Verification items for this drawing (mm, ordinates from the low corner). Coordinates: 2 decimals unless noted, no trailing zeros. Order: outer loops, then holes, each group sorted by start corner. A loop starts at its lowest first (then second) coordinate and runs counter-clockwise, first axis right, second up. Notation, with made-up numbers: M 84.5,-7 L 92.5,-7 A4 ccw 92.5,0 Z; hole C -23,44 d6. An arc over 180 degrees is marked long. Answer as a JSON object with one key per item and string values. Group by question number.
(1) Cross-section at A-A (x = 30). Enter the section's corners in (y, z).
(2) Cross-section at C-C (y = 44). Enter the section's corners in (x, z), plus the area to 3 significant figures.
(3) Gauge pin test, flat ends, axial feed: pin 1 Ø2 at (y, z) = (28.5, 9.5) entering from -X; pin 2 Ø1.5 at (x, y) = (14, 39) entering from -Z; pin 3 Ø4 at (x, z) = (46, 21.5) entering from +Y. Record the tip position at first contact, or that the pin passes through.
(4) Material ranges on line 1 (Y direction, x = 30, z = 45); line 2 (Z direction, x = 50.5, y = 51); line 3 (Y direction, x = 19.5, z = 51) (1 decimal), recorded low to high.
(5) Cross-section at B-B (z = 21.5). Enter the section's corners in (x, y).
(6) Cross-section at D-D (x = 47.5). Enter the section's corners in (y, z) (1 decimal).
(7) Mould release check, pull along Y, two halves, no side actions. Record for the marked faces 1 and 2: released by +Y, released by -Y, zero draft, split by the parting line, or undercut.
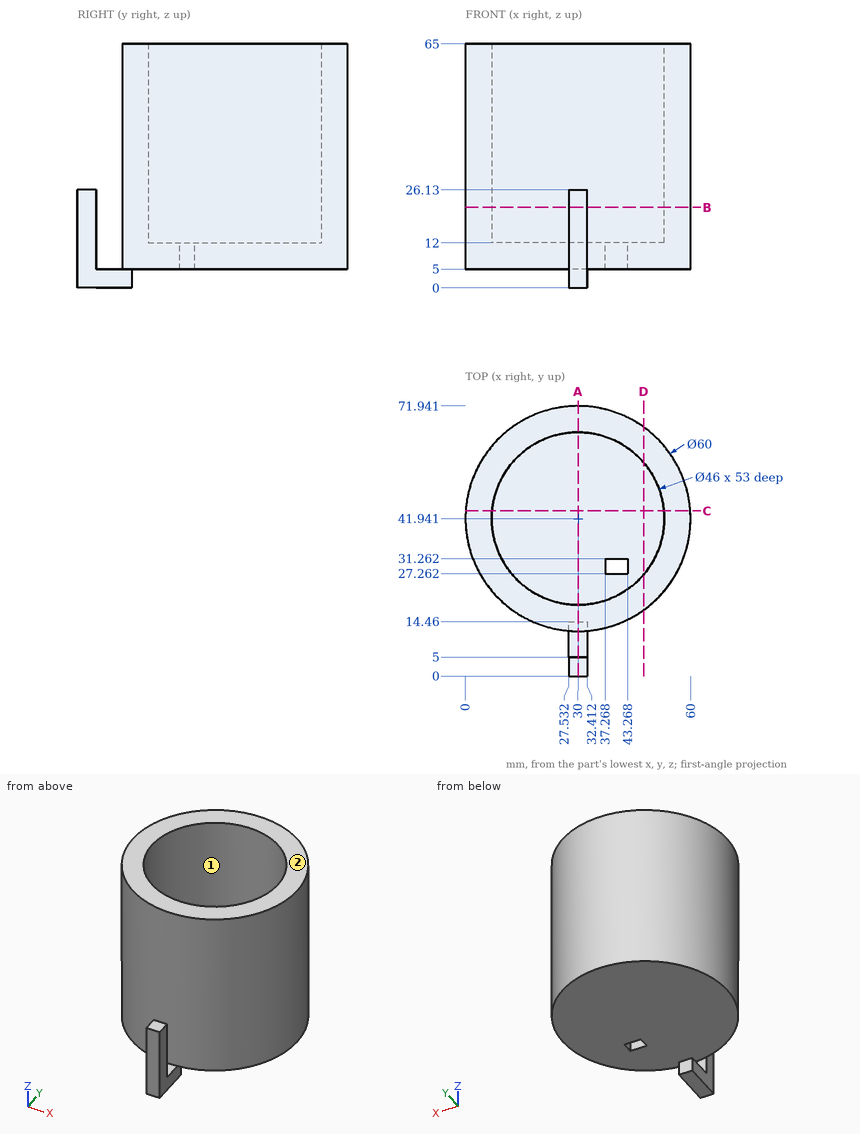
Taken from the geometry:
{
 "1": {"outline": "M 0,0 L 14.46,0 L 14.46,5 L 71.94,5 L 71.94,65 L 64.94,65 L 64.94,12 L 18.94,12 L 18.94,65 L 11.94,65 L 11.94,5 L 5,5 L 5,26.13 L 0,26.13 Z"},
 "2": {"outline": "M 0.07,5 L 59.93,5 L 59.93,65 L 52.91,65 L 52.91,12 L 7.09,12 L 7.09,65 L 0.07,65 Z", "area": "1,160 mm²"},
 "3": {"pin 1": "stops at x = 2.7", "pin 2": "stops at z = 5", "pin 3": "stops at y = 68.47"},
 "4": {"line 1": "y = 11.94 to 18.94, 64.94 to 71.94", "line 2": "z = 5 to 12", "line 3": "y = 13.8 to 21.5, 62.4 to 70"},
 "5": {"outline": "C 30,41.94 d60; M 27.53,0 L 32.41,0 L 32.41,5 L 27.53,5 Z; hole C 30,41.94 d46"},
 "6": {"outline": "M 17.6,5 L 66.3,5 L 66.3,65 L 56.9,65 L 56.9,12 L 27,12 L 27,65 L 17.6,65 Z"},
 "7": {"face 1": "undercut", "face 2": "zero draft"}
}
